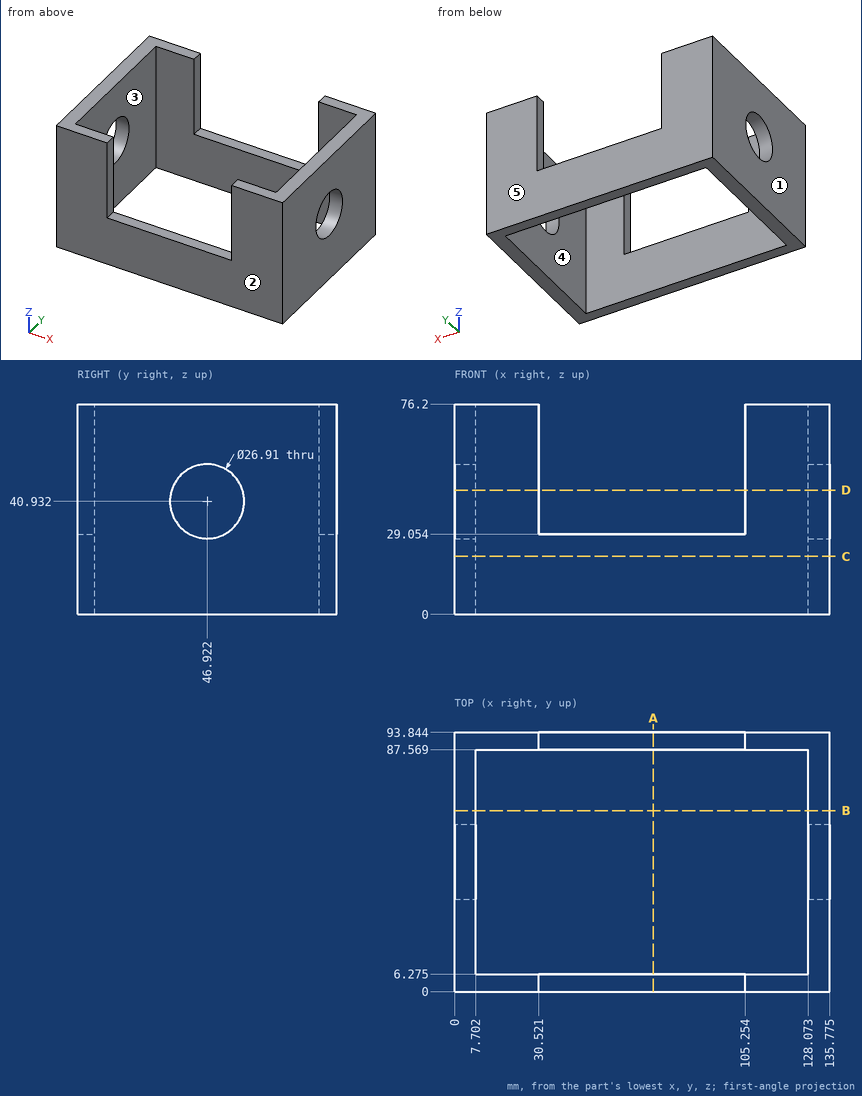
Here's the drawing with two shaded views (mm, measured from the low corner). I have some questions. A direction names the side the tool comes from. Coordinates: 2 decimals unless noted, no trailing zeros. Write each loop counter-clockwise with the first axis right and the second up, starting at its lowest first coordinate (ties: lowest second). Pieces come first, ordered by that corner, then holes. Notation, with made-up numbers: (19, -25.75) -> (77, -25.75) arc R18 cw to (77, -13.75) -> close; hole circle Ø11 at (-33.5, 44.5). An arc over 180 degrees is marked (long way). Use a Markdown table: item, result. Add a question column.
(1) If we section it at D-D, the plane z = 45: Write out the boundary of the cut face in (x, y) (1 decimal), and give its area (3 significant figures).
(2) If we section it at A-A, the plane x = 72: Write out the boundary of the cut face in (y, z) (1 decimal), and give its area (3 significant figures).
(3) Please list where these lines run through material, in increasing order: line 1 (Y direction, x = 16, z = 38) (1 decimal); line 2 (X direction, y = 17, z = 56.5) (1 decimal).
(4) If we section it at B-B, the plane y = 65.5: Write out the boundary of the cut face in (x, z) (1 decimal).
(5) If we section it at C-C, the plane z = 21: Write out the boundary of the cut face in (x, y) (1 decimal).
(6) For the marked faces 4 and 5, which set-ups out of +Z, -Z, +X, -X, +Y, -Y let a thin tool reach every point of the face, with its end or its side?
(7) I'm going to push a flat-ended pin straight in: P1, Ø7, axis at x = 58.5, y = 3, coming from the +Z side. Where does the tip first touch, or does it pass through?
(8) We'd pull the mould along Y, two halves only. Please class the marked faces 1, 2 and 3: +Y half, -Y half, draft (parallel to the pull), parting line (faces both ways), or undercut.
Outcome:
| question | item | result |
|---|---|---|
| 1 | outline | (0, 0) -> (30.5, 0) -> (30.5, 6.3) -> (7.7, 6.3) -> (7.7, 34.1) -> (0, 34.1) -> close; (0, 59.7) -> (7.7, 59.7) -> (7.7, 87.6) -> (30.5, 87.6) -> (30.5, 93.8) -> (0, 93.8) -> close; (105.3, 0) -> (135.8, 0) -> (135.8, 34.1) -> (128.1, 34.1) -> (128.1, 6.3) -> (105.3, 6.3) -> close; (105.3, 87.6) -> (128.1, 87.6) -> (128.1, 59.7) -> (135.8, 59.7) -> (135.8, 93.8) -> (105.3, 93.8) -> close |
| 1 | area | 1,620 mm^2 |
| 2 | outline | (0, 0) -> (6.3, 0) -> (6.3, 29.1) -> (0, 29.1) -> close; (87.6, 0) -> (93.8, 0) -> (93.8, 29.1) -> (87.6, 29.1) -> close |
| 2 | area | 365 mm^2 |
| 3 | line 1 | y = 0 to 6.3, 87.6 to 93.8 |
| 3 | line 2 | x = 0 to 7.7, 128.1 to 135.8 |
| 4 | outline | (0, 0) -> (7.7, 0) -> (7.7, 76.2) -> (0, 76.2) -> close; (128.1, 0) -> (135.8, 0) -> (135.8, 76.2) -> (128.1, 76.2) -> close |
| 5 | outline | (0, 0) -> (135.8, 0) -> (135.8, 93.8) -> (0, 93.8) -> close; hole (7.7, 6.3) -> (128.1, 6.3) -> (128.1, 87.6) -> (7.7, 87.6) -> close |
| 6 | face 4 | +Z, -Z |
| 6 | face 5 | +Z, -Z, +X, -X, +Y |
| 7 | P1 | stops at z = 29.05 |
| 8 | face 1 | draft |
| 8 | face 2 | -Y half |
| 8 | face 3 | undercut |
